Verification items for the finished model (mm, model axes). Face numbers are marked on the shaded views. Round coordinates to 2 decimals unless told otherwise and drop trailing zeros. Write each loop counter-clockwise with the first axis right and the second up, starting at its lowest first coordinate (ties: lowest second). Pieces come first, ordered by that corner, then holes. Notation, with made-up numbers: M -3,81 L 44,81 A16 cw 44,87 Z; hole C -19.75,6.25 d4. An arc over 180 degrees is marked long. Write each question's results on one line, items separated by ' | '.
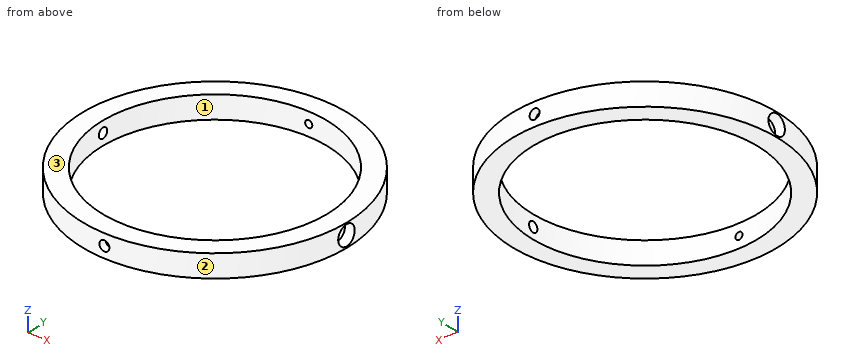
from build123d import *

# Parameters (mm, degrees)
SKETCH1_R           = 42.06875
SKETCH1_R_2         = 35.71875
BOSS_EXTRUDE1_DEPTH = 3.571875
HOLE1_D             = 3.175
HOLE1_DEPTH         = 2.38125
CIRPATTERN1_COUNT   = 2


with BuildPart() as part:
    # Sketch1 → Boss-Extrude1 (new body, symmetric)
    with BuildSketch(Plane.XY):
        Circle(SKETCH1_R)
        Circle(SKETCH1_R_2, mode=Mode.SUBTRACT)
    extrude(amount=BOSS_EXTRUDE1_DEPTH, both=True)

    # Hole1
    with Locations(Plane(origin=(0, 42.06875, 0), x_dir=(1, 0, 0), z_dir=(0, 1, 0))):
        with Locations((0, 0)):
            hole1 = Hole(HOLE1_D / 2, depth=HOLE1_DEPTH)

    # Sketch7 → #4-40 Tapped Hole1 (revolve, cut)
    with BuildSketch(Plane(origin=(0, 39.6875, 0), x_dir=(0, 0, 1), z_dir=(1, 0, 0))):
        Polygon((0, 0), (0, 8.299152758), (1.1303, 7.62), (1.1303, 0), align=None)
    f_4_40_tapped_hole1 = revolve(axis=Axis((0, 46.0375, 0), (0, -1, 0)), mode=Mode.SUBTRACT)

    # Sketch8 → Hole2 (revolve, cut)
    with BuildSketch(Plane(origin=(-42.06875, 0, 0), x_dir=(0, 0, 1), z_dir=(0, 1, 0))):
        Polygon((0, 0), (0, 12.7), (1.5875, 12.7), (1.5875, 4.098342513), (3.1242, 3.175), (3.1242, 0), align=None)
    hole2 = revolve(axis=Axis((-48.198773899, 0, 0), (1, 0, 0)), mode=Mode.SUBTRACT)

    # CirPattern1: Hole1, #4-40 Tapped Hole1, Hole2 ×2 about axis
    cirpattern1_axis = Axis((0, 0, 3.571875), (0, 0, -1))
    for i in range(1, CIRPATTERN1_COUNT):
        add(hole1.rotate(cirpattern1_axis, i * 360 / CIRPATTERN1_COUNT), mode=Mode.SUBTRACT)
        add(f_4_40_tapped_hole1.rotate(cirpattern1_axis, i * 360 / CIRPATTERN1_COUNT), mode=Mode.SUBTRACT)
        add(hole2.rotate(cirpattern1_axis, i * 360 / CIRPATTERN1_COUNT), mode=Mode.SUBTRACT)


solid = part.part
1) Sectioned sample at D-D, the plane x = -33. Record the cut outline in (y, z).
Calculated:
outline: M -26.09,-3.57 L -13.67,-3.57 L -13.67,3.57 L -26.09,3.57 Z; M 13.67,-3.57 L 26.09,-3.57 L 26.09,3.57 L 13.67,3.57 Z
2) Sectioned sample at A-A, the plane x = 0. Record the cut outline in (y, z), and give its area (3 significant figures).
Calculated:
outline: M -42.07,-3.57 L -35.72,-3.57 L -35.72,-1.13 L -39.69,-1.13 L -39.69,-1.59 L -42.07,-1.59 Z; M -42.07,1.59 L -39.69,1.59 L -39.69,1.13 L -35.72,1.13 L -35.72,3.57 L -42.07,3.57 Z; M 35.72,-3.57 L 42.07,-3.57 L 42.07,-1.59 L 39.69,-1.59 L 39.69,-1.13 L 35.72,-1.13 Z; M 35.72,1.13 L 39.69,1.13 L 39.69,1.59 L 42.07,1.59 L 42.07,3.57 L 35.72,3.57 Z | area: 57.7 mm²
3) Sectioned sample at C-C, the plane z = 0. Count the separate pieces of the cut face and the enclosed holes in it, and give its area (3 significant figures).
Calculated:
separate pieces: 4 | enclosed holes: 0 | area: 1,460 mm²
4) Material ranges on line 1 (Z direction, x = 0, y = 37.1); line 2 (X direction, y = 15, z = 3); line 3 (Z direction, x = 0, y = 40.6), recorded low to high. Write a range as [from, to].
Calculated:
line 1: z = [-3.57, -1.13], [1.13, 3.57] | line 2: x = [-39.3, -32.42], [32.42, 39.3] | line 3: z = [-3.57, -1.59], [1.59, 3.57]
5) Depth check by flat-ended pin: P1, Ø3, axis at x = -29, z = 0, coming from the -Y side; P2, Ø3, axis at x = 0, z = 0, coming from the -Y side; P3, Ø2, axis at x = -6.5, z = -0.5, coming from the -Y side. Enter the tip coordinate at first touch or a pass-through.
Calculated:
P1: stops at y = -31.84 | P2: stops at y = -39.69 | P3: stops at y = -41.71
6) Sectioned sample at B-B, the plane y = 0. Record the cut outline in (x, z).
Calculated:
outline: M -42.07,-3.57 L -35.72,-3.57 L -35.72,-1.59 L -37.97,-1.59 L -38.89,-3.12 L -42.07,-3.12 Z; M -42.07,3.12 L -38.89,3.12 L -37.97,1.59 L -35.72,1.59 L -35.72,3.57 L -42.07,3.57 Z; M 35.72,-3.57 L 42.07,-3.57 L 42.07,-3.12 L 38.89,-3.12 L 37.97,-1.59 L 35.72,-1.59 Z; M 35.72,1.59 L 37.97,1.59 L 38.89,3.12 L 42.07,3.12 L 42.07,3.57 L 35.72,3.57 Z
7) Draft check along X on the marked faces 1, 2 and 3. Enter one of: pulls with the +X half, pulls with the -X half, needs draft (parallel to the pull), parting line crosses it, or undercut.
Calculated:
face 1: undercut | face 2: parting line crosses it | face 3: needs draft
